```python
from build123d import *

# Parameters (mm, degrees)
SKETCH1_R                = 13.75
SKETCH1_R_2              = 4.15
BOSS_EXTRUDE1_DEPTH      = 2.5
SKETCH2_R                = 6.5
SKETCH2_R_2              = 4.15
BOSS_EXTRUDE2_DEPTH      = 2.5
CUT_EXTRUDE1_DEPTH       = 21.077973005
FILLET1_R                = 0.5
CIRPATTERN1_COUNT        = 2
FILLET1_OF_CIRPATTERN1_R = 0.5


with BuildPart() as part:
    # Sketch1 → Boss-Extrude1 (new body)
    with BuildSketch(Plane.XY):
        Circle(SKETCH1_R)
        Circle(SKETCH1_R_2, mode=Mode.SUBTRACT)
    extrude(amount=BOSS_EXTRUDE1_DEPTH)

    # Sketch2 → Boss-Extrude2 (add)
    with BuildSketch(Plane.XY.offset(2.5)):
        Circle(SKETCH2_R)
        Circle(SKETCH2_R_2, mode=Mode.SUBTRACT)
    extrude(amount=BOSS_EXTRUDE2_DEPTH)

    # Sketch5 → Cut-Extrude1 (cut, through all)
    with BuildSketch(Plane.XY):
        with BuildLine():
            Line((0, 12.75), (0, 7.5))
            ThreePointArc((0, 7.5), (5.303300859, 5.303300859), (7.5, 0))
            Line((7.5, 0), (12.75, 0))
            ThreePointArc((12.75, 0), (9.01561146, 9.01561146), (0, 12.75))
        make_face()
    cut_extrude1 = extrude(amount=CUT_EXTRUDE1_DEPTH, mode=Mode.SUBTRACT)

    # Fillet1
    fillet1_edges = [part.edges().sort_by_distance(p)[0] for p in [
        (0, 7.5, 1.25),
        (7.5, 0, 1.25),
        (12.75, 0, 1.25),
        (0, 12.75, 1.25),
    ]]
    fillet(fillet1_edges, radius=FILLET1_R)

    # CirPattern1: Cut-Extrude1 ×2 about axis
    cirpattern1_axis = Axis((0, 0, 0), (0, 0, 1))
    for i in range(1, CIRPATTERN1_COUNT):
        add(cut_extrude1.rotate(cirpattern1_axis, i * 360 / CIRPATTERN1_COUNT), mode=Mode.SUBTRACT)

    # Fillet1 of CirPattern1
    fillet1_of_cirpattern1_edges = [part.edges().sort_by_distance(p)[0] for p in [
        (0, -7.5, 1.25),
        (-7.5, 0, 1.25),
        (-12.75, 0, 1.25),
        (0, -12.75, 1.25),
    ]]
    fillet(fillet1_of_cirpattern1_edges, radius=FILLET1_OF_CIRPATTERN1_R)


solid = part.part
```
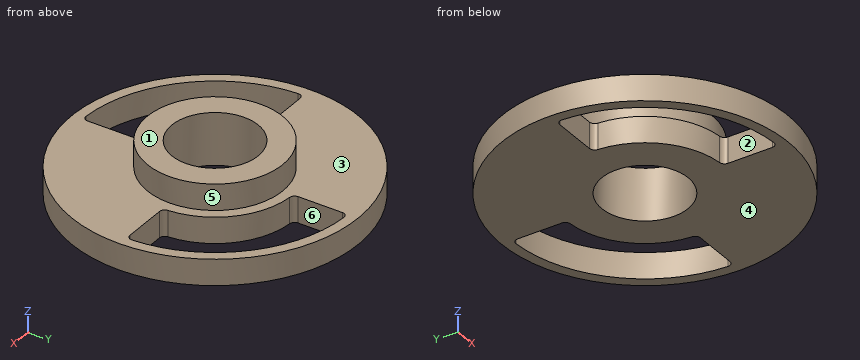
Can you work these out from the model? Positions are in its coordinate system, mm. Face numbers are marked on the shaded views. A direction names the side the tool comes from. Coordinates: 2 decimals unless noted, no trailing zeros. Loops run counter-clockwise (first coordinate to the right, second up) from the corner with the lowest first, then second, coordinate; pieces in that order, holes last. Notation, with made-up numbers: (30, 58.25) - (89, 58.25) arc R6 ccw to (89, 68.25) - close; hole circle Ø6 at (-27.5, 6). An arc over 180 degrees is marked (long way). Use a Markdown table: item, result.
Item 1: I want a section at A-A on z = 2.1. Please give me the cut outline in (x, y), and give its area (3 significant figures).
Numbers:
| item | result |
|---|---|
| outline | circle Ø27.5 at (0, 0); hole (-12.74, -0.52) arc R12.75 ccw to (-0.52, -12.74) arc R0.5 ccw to (0, -12.24) - (0, -7.98) arc R0.5 ccw to (-0.47, -7.49) arc R7.5 cw to (-7.49, -0.47) arc R0.5 ccw to (-7.98, 0) - (-12.24, 0) arc R0.5 ccw to start; hole circle Ø8.3 at (0, 0); hole (0, 7.98) arc R0.5 ccw to (0.47, 7.49) arc R7.5 cw to (7.49, 0.47) arc R0.5 ccw to (7.98, 0) - (12.24, 0) arc R0.5 ccw to (12.74, 0.52) arc R12.75 ccw to (0.52, 12.74) arc R0.5 ccw to (0, 12.24) - close |
| area | 373 mm2 |
Item 2: If I drill on probe 1 along Y at (x, z) = (0, 3.05); probe 2 along X at (y, z) = (-2.75, 1.45); probe 3 along Y at (x, z) = (-0.75, 0.4), over which ranges is the centre line in solid material (lowest first)? Write a range as from..to.
Numbers:
| item | result |
|---|---|
| probe 1 | y = -6.5..-4.15, 4.15..6.5 |
| probe 2 | x = -13.47..-12.45, -6.98..-3.11, 3.11..13.47 |
| probe 3 | y = -13.73..-12.73, -7.46..-4.08, 4.08..13.73 |
Item 3: We'd pull the mould along Y, two halves only. Please class the marked faces 4, 5 and 6: released by +Y, released by -Y, zero draft, split by the parting line, or undercut.
Numbers:
| item | result |
|---|---|
| face 4 | zero draft |
| face 5 | split by the parting line |
| face 6 | undercut |
Item 4: I want a section at B-B on y = 6. Please give me the cut outline in (x, z).
Numbers:
| item | result |
|---|---|
| outline | (-12.37, 0) - (4.5, 0) - (4.5, 2.5) - (2.5, 2.5) - (2.5, 5) - (-2.5, 5) - (-2.5, 2.5) - (-12.37, 2.5) - close; (11.25, 0) - (12.37, 0) - (12.37, 2.5) - (11.25, 2.5) - close |
Item 5: I want a section at D-D on y = -1.5. Please give me the cut outline in (x, z), and give its area (3 significant figures).
Numbers:
| item | result |
|---|---|
| outline | (-13.67, 0) - (-12.66, 0) - (-12.66, 2.5) - (-13.67, 2.5) - close; (-7.35, 0) - (-3.87, 0) - (-3.87, 5) - (-6.32, 5) - (-6.32, 2.5) - (-7.35, 2.5) - close; (3.87, 0) - (13.67, 0) - (13.67, 2.5) - (6.32, 2.5) - (6.32, 5) - (3.87, 5) - close |
| area | 48.0 mm2 |
Item 6: For the marked faces 1, 2 and 3, which set-ups out of +Z, -Z, +X, -X, +Y, -Y let a thin tool reach every point of the face, with its end or its side?
Numbers:
| item | result |
|---|---|
| face 1 | +Z, +X, -X, +Y, -Y |
| face 2 | +Z, -Z |
| face 3 | +Z |
Item 7: Will these pins go through, and if not, where does the flat tip stop? pin 1 (1.2 mm diameter, centred on y = -9.5, z = 1.5, fed in from -X); pin 2 (2 mm diameter, centred on y = -6.5, z = 3, fed in from +X); pin 3 (0.8 mm diameter, centred on x = -11, z = 1, fed in from -Y).
Numbers:
| item | result |
|---|---|
| pin 1 | stops at x = -10.48 |
| pin 2 | stops at x = 12.54 |
| pin 3 | stops at y = -8.76 |
Item 8: I want a section at C-C on x = -7. Please give me the cut outline in (y, z).
Numbers:
| item | result |
|---|---|
| outline | (-11.83, 0) - (-10.66, 0) - (-10.66, 2.5) - (-11.83, 2.5) - close; (-2.69, 0) - (11.83, 0) - (11.83, 2.5) - (-2.69, 2.5) - close |
